Design review of the part built by this model. Coordinates are the model's own, in mm. A direction names the side the tool comes from. Give positions to 0.01 mm unless a question says otherwise; leave off trailing zeros. Loops run counter-clockwise (first coordinate to the right, second up) from the corner with the lowest first, then second, coordinate; pieces in that order, holes last. Notation, with made-up numbers: M 40,-31 L 68,-31 A21 cw 68,-6 Z; hole C 51.25,-23 d9. An arc over 180 degrees is marked long. Answer as CSV lines item,"result".
```python
from build123d import *

# Parameters (mm, degrees)
BOSS_EXTRUDE1_DEPTH = 5
BOSS_EXTRUDE2_DEPTH = 2
FILLET1_R           = 1
FILLET2_R           = 0.2


with BuildPart() as part:
    # Sketch2 → Boss-Extrude1 (new body)
    with BuildSketch(Plane(origin=(0, 0, 0), x_dir=(1, 0, 0), z_dir=(0, 1, 0))):
        Polygon((0, 0), (-2.078460969, 0), (-1.039230485, 1.8), align=None)
    extrude(amount=BOSS_EXTRUDE1_DEPTH)

    # Sketch3 → Boss-Extrude2 (add)
    with BuildSketch(Plane.XZ):
        with BuildLine():
            Line((-4.078460969, 0), (2, 0))
            Line((2, 0), (2, -1))
            ThreePointArc((2, -1), (1.414213562, -2.414213562), (0, -3))
            Line((0, -3), (-2.078460969, -3))
            ThreePointArc((-2.078460969, -3), (-3.492674531, -2.414213562), (-4.078460969, -1))
            Line((-4.078460969, -1), (-4.078460969, 0))
        make_face()
    extrude(amount=BOSS_EXTRUDE2_DEPTH)

    # Fillet1
    fillet1_edges = [part.edges().sort_by_distance(p)[0] for p in [
        (-4.078460969, -2, -0.5),
        (-3.492674531, -2, -2.414213562),
        (-1.039230485, -2, -3),
        (2, -2, -0.5),
        (1.414213562, -2, -2.414213562),
        (-4.078460969, -1, 0),
        (2, -1, 0),
    ]]
    fillet(fillet1_edges, radius=FILLET1_R - 0.0001)  # a hair under: the kernel refuses the full size

    # Fillet2
    fillet2_edges = [part.edges().sort_by_distance(p)[0] for p in [
        (0, 2.5, 0),
        (-2.078460969, 2.5, 0),
        (-1.039230485, 2.5, -1.8),
    ]]
    fillet(fillet2_edges, radius=FILLET2_R)


solid = part.part
```
1. We need section B-B, the plane y = 3.25. Write out the cut boundary in (x, z).
Answer block:
outline,"M -1.91,-0.3 L -1.21,-1.5 A0.2 ccw -0.87,-1.5 L -0.17,-0.3 A0.2 ccw -0.35,0 L -1.73,0 A0.2 ccw Z"
2. We need section A-A, the plane x = -0.75. Write out the cut boundary in (y, z).
Answer block:
outline,"M -2,-2 A1 ccw -1,-3 L 0,-3 L 0,-1.3 L 5,-1.3 L 5,0 L -2,0 Z"
3. We need section C-C, the plane z = -0.45. Write out the cut boundary in (x, y), plus the area to 3 significant figures.
Answer block:
outline,"M -3.91,-1.55 A1 ccw -3.08,-2 L 1,-2 A1 ccw 1.84,-1.55 L 1.84,0 L -0.26,0 L -0.26,5 L -1.82,5 L -1.82,0 L -3.91,0 Z"
area,"19.1 mm²"
4. For faces 1 (the flat face through (-0.524, 2.465, -0.908)), 2 (the flat face through (-1.564, 2.465, -0.892)), 3 (the flat face through (-1, -2, -1)), list the 3-axis set-ups (+Z, -Z, +X, -X, +Y, -Y) from which the entire face can be reached by the end or side of a thin tool; tool diameter is ignored.
Answer block:
face 1,"-Z, +X, +Y"
face 2,"-Z, -X, +Y"
face 3,"+Z, -Z, +X, -X, -Y"
5. For P1, Ø1, axis at y = 1.5, z = -2.5, coming from the -X side; P2, Ø1.5, axis at y = 0, z = -2.5, coming from the -X side, all flat-tipped, find the tip position at first contact; note any pin that passes through.
Answer block:
P1,"through"
P2,"x = -3.93"
6. To check wall thickness, follow L1, parallel to Y at x = 0.5, z = -0.55; L2, parallel to Y at x = -3.5, z = -0.7; L3, parallel to Z at x = -1.5, y = 3.75. State the ranges of each line that lie inside material, in increasing order. Write a range as [from, to].
Answer block:
L1,"[-2, 0]"
L2,"[-1.91, 0]"
L3,"[-1, 0]"
